from build123d import *

# Parameters (mm, degrees)
SKETCH2_W           = 27
SKETCH2_H           = 60
BOSS_EXTRUDE1_DEPTH = 7.5
BOSS_EXTRUDE2_DEPTH = 16.5
SKETCH4_R           = 4
CUT_EXTRUDE1_DEPTH  = 51.222007128
SKETCH5_R           = 3.3
CUT_EXTRUDE2_DEPTH  = 37.803532439


with BuildPart() as part:
    # Sketch2 → Boss-Extrude1 (new body)
    with BuildSketch(Plane(origin=(0, 0, 0), x_dir=(1, 0, 0), z_dir=(0, 1, 0))):
        Rectangle(SKETCH2_W, SKETCH2_H)
    extrude(amount=BOSS_EXTRUDE1_DEPTH)

    # Sketch3 → Boss-Extrude2 (add)
    with BuildSketch(Plane(origin=(0, 7.5, 0), x_dir=(1, 0, 0), z_dir=(0, 1, 0))):
        Polygon((-13.5, -30), (-8.5, -30), (-8.5, -12), (13.5, -12), (13.5, 12), (-8.5, 12), (-8.5, 30), (-13.5, 30), (-13.5, 10), (9.5, 10), (9.5, -10), (-13.5, -10), align=None)
    extrude(amount=BOSS_EXTRUDE2_DEPTH)

    # Sketch4 → Cut-Extrude1 (cut, through all)
    with BuildSketch(Plane.XY.offset(12)):
        with Locations((-3.5, 17)):
            Circle(SKETCH4_R)
    extrude(amount=-CUT_EXTRUDE1_DEPTH, mode=Mode.SUBTRACT)

    # Sketch5 → Cut-Extrude2 (cut, through all)
    with BuildSketch(Plane(origin=(0, 7.5, 0), x_dir=(1, 0, 0), z_dir=(0, 1, 0))):
        with Locations(Location((5.287468246, -21, 0), (0, 0, 270))):
            Circle(SKETCH5_R)
        with Locations(Location((5.287468246, 21, 0), (0, 0, 90))):
            Circle(SKETCH5_R)
    extrude(amount=-CUT_EXTRUDE2_DEPTH, mode=Mode.SUBTRACT)


solid = part.part
Build history of the part. All positions in model axes, mm. A direction names the side the tool comes from. Give positions to 0.01 mm unless a question says otherwise; leave off trailing zeros. Order: outer loops, then holes, each group sorted by start corner. A loop starts at its lowest first (then second) coordinate and runs counter-clockwise, first axis right, second up. Notation, with made-up numbers: M -26,-9 L -8,-9 A18 cw -8,6 Z; hole C -25.5,40 d3. An arc over 180 degrees is marked long. Put each result on its own line as item: value.
Item 1: Two-plate mould, pull along X, no slides. Class faces 4 (the flat face through (-3, 6, -30)), 5 (the flat face through (-8.5, 16, 21)), 6 (the cylindrical face through (8.07, 3.802, 22.774)): +X half, -X half, draft (parallel to the pull), parting line (faces both ways), or undercut.
From the geometry:
face 4: draft
face 5: +X half
face 6: undercut
Item 2: Slice it at D-D, the plane y = 10.75. Write the cut outline in (x, z).
From the geometry:
outline: M -13.5,-30 L -8.5,-30 L -8.5,-12 L 13.5,-12 L 13.5,12 L -8.5,12 L -8.5,30 L -13.5,30 L -13.5,10 L 9.5,10 L 9.5,-10 L -13.5,-10 Z
Item 3: Probe line 1 (Z direction, x = 1, y = 11.75); line 2 (Y direction, x = -3.5, z = -11); line 3 (Z direction, x = 5, y = 6). List the from-to ranges inside material, lowest first. Write a range as [from, to].
From the geometry:
line 1: z = [-12, -10], [10, 12]
line 2: y = [0, 13], [21, 24]
line 3: z = [-30, -24.29], [-17.71, 17.71], [24.29, 30]
Item 4: Slice it at C-C, the plane y = 17. Write the cut outline in (x, z), plus the area to 3 significant figures.
From the geometry:
outline: M -13.5,-30 L -8.5,-30 L -8.5,-12 L -7.5,-12 L -7.5,-10 L -13.5,-10 Z; M -13.5,10 L -7.5,10 L -7.5,12 L -8.5,12 L -8.5,30 L -13.5,30 Z; M 0.5,-12 L 13.5,-12 L 13.5,12 L 0.5,12 L 0.5,10 L 9.5,10 L 9.5,-10 L 0.5,-10 Z
area: 336 mm2
Item 5: 3-axis set-ups, long thin cutter, end or side, ignore diameter. For faces 1 (the flat face through (2, 16, 12)), 2 (the flat face through (0, 14, -10)), 3 (the flat face through (2, 7.5, -19)): which of +Z, -Z, +X, -X, +Y, -Y reach the whole face in a straight line?
From the geometry:
face 1: +Z, +X, +Y
face 2: -X, +Y
face 3: -Z, +X, +Y
Item 6: Flat gauge pins, fed straight in: pin 1 Ø14.5 at (x, z) = (4, -23) entering from +Y; pin 2 Ø4 at (y, z) = (20, 4.5) entering from -X; pin 3 Ø1.5 at (x, y) = (-2.5, 14) entering from -Z; pin 4 Ø8 at (y, z) = (18.5, -23.5) entering from +X. Where does each tip first touch, or does it go through?
From the geometry:
pin 1: stops at y = 7.5
pin 2: stops at x = 9.5
pin 3: passes through
pin 4: stops at x = -8.5
Item 7: Slice it at B-B, the plane z = -21. Write the cut outline in (x, y).
From the geometry:
outline: M -13.5,0 L 1.99,0 L 1.99,7.5 L -8.5,7.5 L -8.5,24 L -13.5,24 Z; M 8.59,0 L 13.5,0 L 13.5,7.5 L 8.59,7.5 Z
Item 8: Slice it at A-A, the plane x = -3.5. Write the cut outline in (y, z).
From the geometry:
outline: M 0,-30 L 7.5,-30 L 7.5,-12 L 13,-12 L 13,-10 L 7.5,-10 L 7.5,10 L 13,10 L 13,12 L 7.5,12 L 7.5,30 L 0,30 Z; M 21,-12 L 24,-12 L 24,-10 L 21,-10 Z; M 21,10 L 24,10 L 24,12 L 21,12 Z
